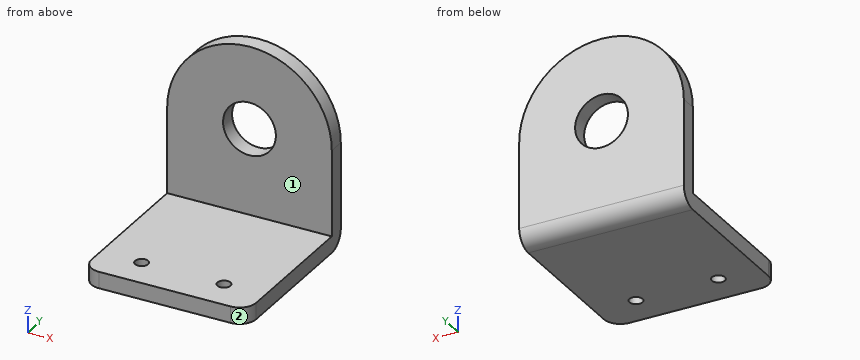
```python
from build123d import *

# Parameters (mm, degrees)
SCHIZZO1_R                           = 8.025
SCHIZZO1_R_2                         = 2
BASE_FLANGIA1_DEPTH                  = 5
PIEGATURA_START                      = -25
PIEGATURA_DELLO_SCHIZZO1_OUTLINE_W   = 50
PIEGATURA_DELLO_SCHIZZO1_OUTLINE_H   = 5
PIEGATURA_DELLO_SCHIZZO1_DEPTH       = 51
PIEGATURA_START_2                    = -30
PIEGATURA_DELLO_SCHIZZO1_2_OUTLINE_R = 8.025
PIEGATURA_DELLO_SCHIZZO1_2_DEPTH     = 5
PIEGATURA_START_3                    = -26
PIEGATURA_DELLO_SCHIZZO1_3_DEPTH     = 51
PIEGATURA_DELLO_SCHIZZO1_4_DEPTH     = 50


with BuildPart() as part:
    # Base-Flangia1: sheet metal written as solids
    # Schizzo1 → Base-Flangia1 (new body)
    with BuildSketch(Plane.XY):
        with BuildLine():
            Line((-25, -72), (-25, 0))
            ThreePointArc((-25, 0), (0, 25), (25, 0))
            Line((25, 0), (25, -72))
            ThreePointArc((25, -72), (23.535533906, -75.535533906), (20, -77))
            Line((20, -77), (-20, -77))
            ThreePointArc((-20, -77), (-23.535533906, -75.535533906), (-25, -72))
        make_face()
        Circle(SCHIZZO1_R, mode=Mode.SUBTRACT)
        with Locations((-12.5, -67)):
            Circle(SCHIZZO1_R_2, mode=Mode.SUBTRACT)
        with Locations((12.5, -67)):
            Circle(SCHIZZO1_R_2, mode=Mode.SUBTRACT)
    extrude(amount=-BASE_FLANGIA1_DEPTH)

    # Piegatura dello schizzo1: read off the stored shape, not the designer's step
    # Piegatura dello schizzo1 outline → Piegatura dello schizzo1 (cut)
    with BuildSketch(Plane(origin=(0, 0, 0), x_dir=(1, 0, 0), z_dir=(0, 1, 0)).offset(PIEGATURA_START)):
        with Locations((0, 2.5)):
            Rectangle(PIEGATURA_DELLO_SCHIZZO1_OUTLINE_W, PIEGATURA_DELLO_SCHIZZO1_OUTLINE_H)
    extrude(amount=PIEGATURA_DELLO_SCHIZZO1_DEPTH, mode=Mode.SUBTRACT)

    # Piegatura dello schizzo1 2 outline → Piegatura dello schizzo1 2 (add)
    with BuildSketch(Plane(origin=(0, 0, 0), x_dir=(1, 0, 0), z_dir=(0, 1, 0)).offset(PIEGATURA_START_2)):
        with BuildLine():
            Line((-25, 0), (-25, -26.07730122))
            ThreePointArc((-25, -26.07730122), (0, -51.07730122), (25, -26.07730122))
            Line((25, -26.07730122), (25, 0))
            Line((25, 0), (-25, 0))
        make_face()
        with Locations((0, -26.07730122)):
            Circle(PIEGATURA_DELLO_SCHIZZO1_2_OUTLINE_R, mode=Mode.SUBTRACT)
    extrude(amount=PIEGATURA_DELLO_SCHIZZO1_2_DEPTH)

    # Piegatura dello schizzo1 3 outline → Piegatura dello schizzo1 3 (cut)
    with BuildSketch(Plane.YZ.offset(PIEGATURA_START_3)):
        with BuildLine():
            ThreePointArc((-25, 0.01), (-26.467395026, -3.532604974), (-30.01, -5))
            Line((-30.01, -5), (-25, -5))
            Line((-25, -5), (-25, 0.01))
        make_face()
    extrude(amount=PIEGATURA_DELLO_SCHIZZO1_3_DEPTH, mode=Mode.SUBTRACT)

    # Piegatura dello schizzo1 4 outline → Piegatura dello schizzo1 4 (add)
    with BuildSketch(Plane.YZ.offset(PIEGATURA_START)):
        with BuildLine():
            ThreePointArc((-30, 0.01), (-30.002928932, 0.002928932), (-30.01, 0))
            Line((-30.01, 0), (-30, 0))
            Line((-30, 0), (-30, 0.01))
        make_face()
    extrude(amount=PIEGATURA_DELLO_SCHIZZO1_4_DEPTH)


solid = part.part
```
CAD build for the part. Positions are in the model's coordinates, mm. Face numbers are marked on the shaded views. A direction names the side the tool comes from. Round coordinates to 2 decimals unless told otherwise and drop trailing zeros. Order: outer loops, then holes, each group sorted by start corner. A loop starts at its lowest first (then second) coordinate and runs counter-clockwise, first axis right, second up. Notation, with made-up numbers: (44, 68) - (48, 68) arc R17 ccw to (48, 90) - close; hole circle Ø8 at (29.25, 57.5). An arc over 180 degrees is marked (long way). Use CSV: the item, a comma, the result in double quotes. Start each with the question number.
1) Tool access for the marked faces 1 and 2: list every direction of +Z, -Z, +X, -X, +Y, -Y with a clear straight run to the whole face (end or side of a thin tool).
2) Wall check: L1, parallel to Z at x = -20.5, y = -57; L2, parallel to Y at x = 20.5, z = 23; L3, parallel to Y at x = 12.5, z = -1.9. Give the ranges that are in metal, low to high. Write a range as [from, to].
3) Saw through at B-B (y = -67). List the corners of the cut face in (x, z), and give its area (3 significant figures).
4) Pin check, flat tips, straight feed: pin 1 Ø1 at (x, y) = (5.5, -64) entering from +Z; pin 2 Ø10 at (x, z) = (-16, 45) entering from -Y. Stop position of each tip, or through.
5) Saw through at D-D (z = 11.5). List the corners of the cut face in (x, y).
Values follow:
1,face 1,"+Z, +X, -X, -Y"
1,face 2,"+Z, -Z, +X, -Y"
2,L1,"z = [-5, 0]"
2,L2,"y = [-30, -25]"
2,L3,"y = [-77, -69], [-65, -25.38]"
3,outline,"(-25, -5) - (-14.5, -5) - (-14.5, 0) - (-25, 0) - close; (-10.5, -5) - (10.5, -5) - (10.5, 0) - (-10.5, 0) - close; (14.5, -5) - (25, -5) - (25, 0) - (14.5, 0) - close"
3,area,"210 mm2"
4,pin 1,"stops at z = 0"
4,pin 2,"stops at y = -30"
5,outline,"(-25, -30) - (25, -30) - (25, -25) - (-25, -25) - close"
